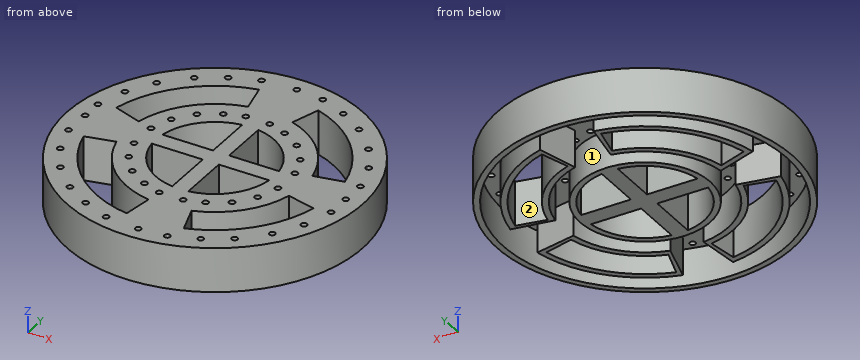
```python
from build123d import *

# Parameters (mm, degrees)
SKETCH1_R           = 127
BOSS_EXTRUDE1_DEPTH = 38.1
SKETCH2_R           = 121.825159098
SKETCH2_R_2         = 55.948426771
CUT_EXTRUDE1_DEPTH  = 31.75
SKETCH4_R           = 2.54
CUT_EXTRUDE3_DEPTH  = 25.4


with BuildPart() as part:
    # Sketch1 → Boss-Extrude1 (new body)
    with BuildSketch(Plane.XY):
        with Locations(Location((-33.762487444, 46.957799842, 0), (0, 0, 180))):
            Circle(SKETCH1_R)
        with BuildLine():
            Line((-26.585000486, -3.332593683), (-26.585000486, 40.517010102))
            Line((-26.585000486, 40.517010102), (16.627553511, 40.517010102))
            ThreePointArc((16.627553511, 40.517010102), (2.420409144, 11.300570639), (-26.585000486, -3.332593683))
        make_face(mode=Mode.SUBTRACT)
        with BuildLine():
            Line((-40.39467032, -3.407407894), (-40.39467032, 40.517010102))
            Line((-40.39467032, 40.517010102), (-84.1525284, 40.517010102))
            ThreePointArc((-84.1525284, 40.517010102), (-69.751682027, 11.105075075), (-40.39467032, -3.407407894))
        make_face(mode=Mode.SUBTRACT)
        with BuildLine():
            Line((65.080698845, 23.450683386), (40.369902273, 29.3274625))
            ThreePointArc((40.369902273, 29.3274625), (22.152677736, -4.81028205), (-10.482872263, -25.599071073))
            Line((-10.482872263, -25.599071073), (-2.723000536, -49.784694711))
            ThreePointArc((-2.723000536, -49.784694711), (40.79106613, -22.066309347), (65.080698845, 23.450683386))
        make_face(mode=Mode.SUBTRACT)
        with BuildLine():
            Line((65.768603115, 67.356868745), (40.885830475, 62.25710152))
            ThreePointArc((40.885830475, 62.25710152), (22.956797892, 97.843580478), (-10.482872263, 119.514670757))
            Line((-10.482872263, 119.514670757), (-2.723000536, 143.700294396))
            ThreePointArc((-2.723000536, 143.700294396), (41.863226338, 114.805507356), (65.768603115, 67.356868745))
        make_face(mode=Mode.SUBTRACT)
        with BuildLine():
            Line((-107.894877162, 29.3274625), (-132.605673734, 23.450683386))
            ThreePointArc((-132.605673734, 23.450683386), (-102.864783632, -27.523289446), (-49.80854646, -53.367092333))
            Line((-49.80854646, -53.367092333), (-45.797031706, -28.28586929))
            ThreePointArc((-45.797031706, -28.28586929), (-85.589209585, -8.903017124), (-107.894877162, 29.3274625))
        make_face(mode=Mode.SUBTRACT)
        with BuildLine():
            Line((16.34326948, 55.327574216), (-26.585000486, 55.327574216))
            Line((-26.585000486, 55.327574216), (-26.585000486, 97.248193368))
            ThreePointArc((-26.585000486, 97.248193368), (1.729442412, 83.302853358), (16.34326948, 55.327574216))
        make_face(mode=Mode.SUBTRACT)
        with BuildLine():
            Line((-108.410805364, 62.25710152), (-132.605673734, 70.464916298))
            ThreePointArc((-132.605673734, 70.464916298), (-104.834687001, 119.561535628), (-55.157232799, 146.27962459))
            Line((-55.157232799, 146.27962459), (-49.80854646, 121.449168403))
            ThreePointArc((-49.80854646, 121.449168403), (-87.913135616, 100.568874282), (-108.410805364, 62.25710152))
        make_face(mode=Mode.SUBTRACT)
        with BuildLine():
            Line((-40.39467032, 55.327574216), (-83.868244368, 55.327574216))
            ThreePointArc((-83.868244368, 55.327574216), (-69.056999185, 83.494595556), (-40.39467032, 97.323007578))
            Line((-40.39467032, 97.323007578), (-40.39467032, 55.327574216))
        make_face(mode=Mode.SUBTRACT)
    extrude(amount=BOSS_EXTRUDE1_DEPTH)

    # Sketch2 → Cut-Extrude1 (cut)
    with BuildSketch(Plane(origin=(0, 0, 0), x_dir=(-1, 0, 0), z_dir=(0, 0, -1))):
        with Locations((33.762487444, 46.957799842)):
            Circle(SKETCH2_R)
        with Locations((33.762487444, 46.957799842)):
            Circle(SKETCH2_R_2, mode=Mode.SUBTRACT)
        with BuildLine():
            Line((138.519360461, 26.640882165), (103.545749119, 33.423787783))
            ThreePointArc((103.545749119, 33.423787783), (82.09047925, -5.169719765), (41.986549655, -23.648417258))
            Line((41.986549655, -23.648417258), (46.108242286, -59.03447311))
            ThreePointArc((46.108242286, -59.03447311), (106.311250274, -31.294718328), (138.519360461, 26.640882165))
        make_face(mode=Mode.SUBTRACT)
        with BuildLine():
            Line((138.519360461, 67.274717519), (104.257428362, 56.086676957))
            ThreePointArc((104.257428362, 56.086676957), (85.1635344, 96.057753653), (46.108242286, 116.961052837))
            Line((46.108242286, 116.961052837), (52.295623345, 152.044918281))
            ThreePointArc((52.295623345, 152.044918281), (108.572936641, 123.051007681), (138.519360461, 67.274717519))
        make_face(mode=Mode.SUBTRACT)
        with BuildLine():
            Line((4.921540725, -55.779629464), (14.550236506, -21.480219608))
            ThreePointArc((14.550236506, -21.480219608), (-18.521954058, -1.200379828), (-36.02077423, 33.423787783))
            Line((-36.02077423, 33.423787783), (-70.994385572, 26.640882165))
            ThreePointArc((-70.994385572, 26.640882165), (-44.725597918, -25.336045292), (4.921540725, -55.779629464))
        make_face(mode=Mode.SUBTRACT)
        with BuildLine():
            Line((-71.448904325, 64.771913071), (-36.323549601, 58.824581363))
            ThreePointArc((-36.323549601, 58.824581363), (-19.092240815, 94.489376641), (14.550236506, 115.395819293))
            Line((14.550236506, 115.395819293), (4.921540725, 149.695229149))
            ThreePointArc((4.921540725, 149.695229149), (-45.58169802, 118.311004544), (-71.448904325, 64.771913071))
        make_face(mode=Mode.SUBTRACT)
    extrude(amount=-CUT_EXTRUDE1_DEPTH, mode=Mode.SUBTRACT)

    # Sketch4 → Cut-Extrude3 (cut)
    with BuildSketch(Plane(origin=(0, 0, 31.75), x_dir=(-1, 0, 0), z_dir=(0, 0, -1))):
        with Locations((31.281297081, -67.505404389)):
            Circle(SKETCH4_R)
        with Locations((60.205260923, -65.29342847)):
            Circle(SKETCH4_R)
        with Locations((83.413284725, -56.002203895)):
            Circle(SKETCH4_R)
        with Locations((104.747838674, -42.951403951)):
            Circle(SKETCH4_R)
        with Locations((124.996169025, -22.689001677)):
            Circle(SKETCH4_R)
        with Locations((138.681871495, 0)):
            Circle(SKETCH4_R)
        with Locations((146.743625587, 25.43589811)):
            Circle(SKETCH4_R)
        with Locations((146.743625587, 49.259285421)):
            Circle(SKETCH4_R)
        with Locations(Location((-27.958558869, 34.347513636, 0), (0, 0, 180))):
            Circle(SKETCH4_R)
        with Locations((44.169136825, -15.737345855)):
            Circle(SKETCH4_R)
        with Locations((60.205260923, -10.25450455)):
            Circle(SKETCH4_R)
        with Locations((76.793334998, 0)):
            Circle(SKETCH4_R)
        with Locations((89.338680519, 15.902012931)):
            Circle(SKETCH4_R)
        with Locations((95.775347578, 34.347513636)):
            Circle(SKETCH4_R)
        with Locations(Location((-21.52189181, 15.902012931, 0), (0, 0, 180))):
            Circle(SKETCH4_R)
        with Locations(Location((-8.976546288, 0, 0), (0, 0, 180))):
            Circle(SKETCH4_R)
        with Locations(Location((7.611527786, -10.25450455, 0), (0, 0, 180))):
            Circle(SKETCH4_R)
        with Locations(Location((23.647651884, -15.737345855, 0), (0, 0, 180))):
            Circle(SKETCH4_R)
        with Locations(Location((-78.926836877, 46.526134027, 0), (0, 0, 180))):
            Circle(SKETCH4_R)
        with Locations(Location((-78.926836877, 25.43589811, 0), (0, 0, 180))):
            Circle(SKETCH4_R)
        with Locations(Location((-70.865082786, 0, 0), (0, 0, 180))):
            Circle(SKETCH4_R)
        with Locations(Location((-57.179380316, -22.689001677, 0), (0, 0, 180))):
            Circle(SKETCH4_R)
        with Locations(Location((-36.931049965, -42.951403951, 0), (0, 0, 180))):
            Circle(SKETCH4_R)
        with Locations(Location((-15.596496015, -56.002203895, 0), (0, 0, 180))):
            Circle(SKETCH4_R)
        with Locations(Location((7.611527786, -65.29342847, 0), (0, 0, 180))):
            Circle(SKETCH4_R)
        with Locations(Location((95.775347578, 58.704754417, 0), (0, 0, 180))):
            Circle(SKETCH4_R)
        with Locations((-27.958558869, 58.704754417)):
            Circle(SKETCH4_R)
        with Locations((-78.926836877, 67.616369944)):
            Circle(SKETCH4_R)
        with Locations((7.611527786, 158.345696523)):
            Circle(SKETCH4_R)
        with Locations((-15.596496015, 149.054471948)):
            Circle(SKETCH4_R)
        with Locations((-36.931049965, 136.003672004)):
            Circle(SKETCH4_R)
        with Locations((-57.179380316, 115.74126973)):
            Circle(SKETCH4_R)
        with Locations((-70.865082786, 93.052268053)):
            Circle(SKETCH4_R)
        with Locations((23.647651884, 108.789613908)):
            Circle(SKETCH4_R)
        with Locations((7.611527786, 103.306772603)):
            Circle(SKETCH4_R)
        with Locations((-8.976546288, 93.052268053)):
            Circle(SKETCH4_R)
        with Locations((-21.52189181, 77.150255122)):
            Circle(SKETCH4_R)
        with Locations(Location((89.338680519, 77.150255122, 0), (0, 0, 180))):
            Circle(SKETCH4_R)
        with Locations(Location((76.793334998, 93.052268053, 0), (0, 0, 180))):
            Circle(SKETCH4_R)
        with Locations(Location((60.205260923, 103.306772603, 0), (0, 0, 180))):
            Circle(SKETCH4_R)
        with Locations(Location((44.169136825, 108.789613908, 0), (0, 0, 180))):
            Circle(SKETCH4_R)
        with Locations(Location((146.743625587, 67.616369944, 0), (0, 0, 180))):
            Circle(SKETCH4_R)
        with Locations(Location((138.681871495, 93.052268053, 0), (0, 0, 180))):
            Circle(SKETCH4_R)
        with Locations(Location((124.996169025, 115.74126973, 0), (0, 0, 180))):
            Circle(SKETCH4_R)
        with Locations(Location((104.747838674, 136.003672004, 0), (0, 0, 180))):
            Circle(SKETCH4_R)
        with Locations(Location((83.413284725, 149.054471948, 0), (0, 0, 180))):
            Circle(SKETCH4_R)
        with Locations(Location((60.205260923, 158.345696523, 0), (0, 0, 180))):
            Circle(SKETCH4_R)
        with Locations(Location((31.281297081, 160.557672442, 0), (0, 0, 180))):
            Circle(SKETCH4_R)
    extrude(amount=-CUT_EXTRUDE3_DEPTH, mode=Mode.SUBTRACT)


solid = part.part
```
Design review of the part built by this model. Coordinates are the model's own, in mm. Face numbers are marked on the shaded views. A direction names the side the tool comes from. Coordinates: 2 decimals unless noted, no trailing zeros. Order: outer loops, then holes, each group sorted by start corner. A loop starts at its lowest first (then second) coordinate and runs counter-clockwise, first axis right, second up. Notation, with made-up numbers: (51, -9.5) - (77, -9.5) arc R16 ccw to (77, -5.5) - close; hole circle Ø5 at (-38.5, 52). An arc over 180 degrees is marked (long way). Answer in a Markdown table with one row per item.
(1) Wall thickness on line 1 along X through (y, z) = (-44.5, 20.5); line 2 along X through (y, z) = (-30, 33.5); line 3 along Y through (x, z) = (-113.5, 2.5): over which ranges is each line inside the solid? List them lowest first. Write a range as from..to.
Checked values:
| item | result |
|---|---|
| line 1 | -121.88..-114.24, -88.74..-78.01, -48.39..-44.42, -8.09..-4.42, 10.49..21.21, 46.72..54.35 |
| line 2 | -134.79..-100.1, -46.07..-9.07, 32.57..67.26 |
| line 3 | -51.89..-45.15, -23.96..-16.01, 27.99..31.49, 59.1..63.98, 109.92..117.87, 139.06..145.81 |
(2) Consider section B-B on z = 5. Give the number of separate pieces and of enclosed holes in the cut face, plus the area to 3 significant figures.
Checked values:
| item | result |
|---|---|
| separate pieces | 6 |
| enclosed holes | 9 |
| area | 13,500 mm^2 |
(3) Clearance check with flat-ended pins moving along their axes: pin 1 (6.5 mm diameter, centred on x = 27.96, y = 34.35, fed in from -Z); pin 2 (11.5 mm diameter, centred on y = 9.5, z = 12, fed in from +X); pin 3 (8 mm diameter, centred on y = 143, z = 16, fed in from +X). State where each tip first meets the part, or that it passes through.
Checked values:
| item | result |
|---|---|
| pin 1 | z = 31.75 |
| pin 2 | x = 89.22 |
| pin 3 | x = 53.74 |
(4) Consider section A-A on y = -33. State the section outline as (x, z) points, plus the area to 3 significant figures.
Checked values:
| item | result |
|---|---|
| outline | (-132.43, 0) - (-125.68, 0) - (-125.68, 31.75) - (-104.43, 31.75) - (-104.43, 0) - (-96.45, 0) - (-96.45, 38.1) - (-132.43, 38.1) - close; (-46.55, 0) - (-43.08, 0) - (-43.08, 31.75) - (-11.32, 31.75) - (-11.32, 0) - (-8.11, 0) - (-8.11, 38.1) - (-46.55, 38.1) - close; (28.92, 0) - (36.9, 0) - (36.9, 31.75) - (58.15, 31.75) - (58.15, 0) - (64.91, 0) - (64.91, 38.1) - (28.92, 38.1) - close |
| area | 1,850 mm^2 |
(5) For the marked faces 1 and 2, list the 3-axis set-ups (+Z, -Z, +X, -X, +Y, -Y) from which the entire face can be reached by the end or side of a thin tool; tool diameter is ignored.
Checked values:
| item | result |
|---|---|
| face 1 | -Z |
| face 2 | +Z, -Z |
